Check sheet for the modelled part. Datum: model origin and axes. Units: mm. Give positions to 0.01 mm unless a question says otherwise; leave off trailing zeros. Write each loop counter-clockwise with the first axis right and the second up, starting at its lowest first coordinate (ties: lowest second). Pieces come first, ordered by that corner, then holes. Notation, with made-up numbers: M 37,22.5 L 59,22.5 A23 ccw 59,50.5 Z; hole C 40.25,44.25 d5. An arc over 180 degrees is marked long. Use CSV: the item, a comma, the result in double quotes. Start each with the question number.
1. Depth check by flat-ended pin: P1, Ø1.5, axis at x = 191, y = 60.5, coming from the +Z side; P2, Ø0.6, axis at y = 60.5, z = 1, coming from the -X side; P3, Ø3, axis at x = 159, y = 116, coming from the +Z side. Enter the tip coordinate at first touch or a pass-through.
2. Scan lines: line 1 (Y direction, x = 191, z = 1.05); line 2 (Z direction, x = 170, y = 144); line 3 (Y direction, x = 189.5, z = 0.95). Record each from-to range of solid material in increasing order.
3. Cross-section at C-C, the plane x = 163. Enter the section's corners in (y, z).
4. Cross-section at A-A, the plane z = 1. Enter the section's corners in (x, y), and give its area (3 significant figures).
5. Cross-section at B-B, the plane y = 149.5. Enter the section's corners in (x, z).
from build123d import *

# Parameters (mm, degrees)
ESQUISSE1_W             = 2.725699057
ESQUISSE1_H             = 2.506306443
BOSS_EXTRU_1_DEPTH      = 0.2
ESQUISSE2_W             = 3.234923292
ESQUISSE2_H             = 9.478551462
BOSS_EXTRU_2_DEPTH      = 1.25
ESQUISSE3_W             = 1.880186225
ESQUISSE3_H             = 7.770248285
ENL_V_MAT_EXTRU_1_DEPTH = 0.75
CONG_1_R                = 1


with BuildPart() as part:
    # Esquisse1 → Boss.-Extru.1 (new body)
    with BuildSketch(Plane.XY):
        with BuildLine():
            Line((126.422039537, 160.93295612), (170.054893457, 160.93295612))
            Line((170.054893457, 160.93295612), (170.054893457, 158.48132271))
            Line((170.054893457, 158.48132271), (178.126916218, 158.48132271))
            Line((178.126916218, 158.48132271), (178.126916218, 144.756393673))
            Line((178.126916218, 144.756393673), (171.779679926, 144.756393673))
            Line((171.779679926, 144.756393673), (170.514624307, 143.320028439))
            Line((170.514624307, 143.320028439), (170.819971895, 71.257993621))
            ThreePointArc((170.819971895, 71.257993621), (171.74909254, 68.47783045), (174.09562451, 66.721026494))
            Line((174.09562451, 66.721026494), (193.829857273, 66.721026494))
            Line((193.829857273, 66.721026494), (193.829857273, 54.476275086))
            Line((193.829857273, 54.476275086), (166.335216501, 54.476275086))
            ThreePointArc((166.335216501, 54.476275086), (158.91775161, 58.528592216), (155.831660909, 66.397270867))
            Line((155.831660909, 66.397270867), (155.831660909, 142.383251424))
            ThreePointArc((155.831660909, 142.383251424), (155.025193292, 143.979631476), (153.414150222, 144.756393673))
            Line((153.414150222, 144.756393673), (123.308343674, 144.756393673))
            Line((123.308343674, 144.756393673), (123.308343674, 158.075350221))
            Line((123.308343674, 158.075350221), (126.422039537, 158.075350221))
            Line((126.422039537, 158.075350221), (126.422039537, 160.93295612))
        make_face()
        with Locations((130.26793419, 159.328503442)):
            Rectangle(ESQUISSE1_W, ESQUISSE1_H, mode=Mode.SUBTRACT)
    extrude(amount=BOSS_EXTRU_1_DEPTH)

    # Esquisse2 → Boss.-Extru.2 (add)
    with BuildSketch(Plane.XY.offset(0.2)):
        with Locations((191.04638423, 60.711911726)):
            Rectangle(ESQUISSE2_W, ESQUISSE2_H)
    extrude(amount=BOSS_EXTRU_2_DEPTH)

    # Esquisse3 → Enlèv. mat.-Extru.1 (cut)
    with BuildSketch(Plane.XY.offset(1.45)):
        with Locations((191.008183709, 60.791242391)):
            Rectangle(ESQUISSE3_W, ESQUISSE3_H)
    extrude(amount=-ENL_V_MAT_EXTRU_1_DEPTH, mode=Mode.SUBTRACT)

    # Congé1
    cong_1_edges = [part.edges().sort_by_distance(p)[0] for p in [
        (193.829857273, 66.721026494, 0.1),
        (193.829857273, 54.476275086, 0.1),
    ]]
    fillet(cong_1_edges, radius=CONG_1_R)


solid = part.part
Worked answers:
1,P1,"stops at z = 0.7"
1,P2,"stops at x = 189.43"
1,P3,"stops at z = 0.2"
2,line 1,"y = 55.97 to 56.91, 64.68 to 65.45"
2,line 2,"z = 0 to 0.2"
2,line 3,"y = 55.97 to 65.45"
3,outline,"M 55.48,0 L 160.93,0 L 160.93,0.2 L 55.48,0.2 Z"
4,outline,"M 189.43,55.97 L 192.66,55.97 L 192.66,65.45 L 189.43,65.45 Z; hole M 190.07,56.91 L 191.95,56.91 L 191.95,64.68 L 190.07,64.68 Z"
4,area,"16.1 mm^2"
5,outline,"M 123.31,0 L 178.13,0 L 178.13,0.2 L 123.31,0.2 Z"
